Design review of the part built by this model. Coordinates are the model's own, in mm. Face numbers are marked on the shaded views. A direction names the side the tool comes from. Round coordinates to 2 decimals unless told otherwise and drop trailing zeros. Loops run counter-clockwise (first coordinate to the right, second up) from the corner with the lowest first, then second, coordinate; pieces in that order, holes last. Notation, with made-up numbers: M 22,51 L 30,51 A37 cw 30,88 Z; hole C -6.5,4.5 d4. An arc over 180 degrees is marked long. One line per item, written item: value. Start each with the question number.
Item 1: We need section B-B (x = 10.72). Write out the cut boundary in (y, z).
Item 2: Clearance check with flat-ended pins moving along their axes: pin 1 (0.8 mm diameter, centred on y = 20, z = 5, fed in from +X); pin 2 (2 mm diameter, centred on y = 20, z = 5, fed in from -X); pin 3 (6 mm diameter, centred on x = 35.5, y = 26, fed in from +Z). State where each tip first meets the part, or that it passes through.
Item 3: Mouldability with a two-part tool opening along Y and no side actions: class the marked faces 1, 2 and 3 as released by +Y, released by -Y, zero draft, split by the parting line, or undercut.
Item 4: For the marked faces 4 and 5, list the 3-axis set-ups (+Z, -Z, +X, -X, +Y, -Y) from which the entire face can be reached by the end or side of a thin tool; tool diameter is ignored.
Item 5: For line 1 along Y through (x, z) = (27.5, 6.9); line 2 along X through (y, z) = (5.5, 4.95); line 3 along Y through (x, z) = (52.5, 4.75), list the stretches that pass through material, from the lowest coordinate up.
Item 6: We need section A-A (y = 48). Write out the cut boundary in (x, z).
from build123d import *

# Parameters (mm, degrees)
SKETCH_W        = 55
SKETCH_H        = 75.8
PAD_DEPTH       = 3.6
SKETCH001_W     = 51.76
SKETCH001_H     = 74.18
PAD001_DEPTH    = 5
POCKET_DEPTH    = 7
SKETCH003_R     = 2
PAD002_DEPTH    = 7.25
SKETCH004_W     = 10
SKETCH004_H     = 2.5
POCKET001_DEPTH = 1
SKETCH005_W     = 10
SKETCH005_H     = 2.5
POCKET002_DEPTH = 1
POCKET003_DEPTH = 2.3
SKETCH007_R     = 1.6
POCKET004_DEPTH = 6.551
CHAMFER_SIZE    = 5
CHAMFER001_SIZE = 2
CHAMFER002_SIZE = 1
CHAMFER003_SIZE = 1
CHAMFER004_SIZE = 1
FILLET_R        = 3
CHAMFER005_SIZE = 0.5
CHAMFER006_SIZE = 1


with BuildPart() as part:
    # Sketch → Pad (new body)
    with BuildSketch(Plane.XY):
        with Locations((27.5, 37.9)):
            Rectangle(SKETCH_W, SKETCH_H)
    extrude(amount=PAD_DEPTH)

    # Sketch001 → Pad001 (new body)
    with BuildSketch(Plane.XY.offset(3.6)):
        with Locations((27.5, 37.09)):
            Rectangle(SKETCH001_W, SKETCH001_H)
    extrude(amount=PAD001_DEPTH)

    # Sketch002 → Pocket (cut)
    with BuildSketch(Plane.XY.offset(8.6)):
        Polygon((18.22, 1.6), (3.22, 1.6), (3.22, 72.58), (51.78, 72.58), (51.78, 1.6), (36.78, 1.6), (36.78, 14.1), (18.22, 14.1), align=None)
    extrude(amount=-POCKET_DEPTH, mode=Mode.SUBTRACT)

    # Sketch003 → Pad002 (new body)
    with BuildSketch(Plane.XY.offset(1.6)):
        with Locations((10.72, 52.58)):
            Circle(SKETCH003_R)
        with Locations((44.28, 52.58)):
            Circle(SKETCH003_R)
        with Locations((18.22, 18.6)):
            Circle(SKETCH003_R)
        with Locations((36.78, 18.6)):
            Circle(SKETCH003_R)
    extrude(amount=PAD002_DEPTH)

    # Sketch004 → Pocket001 (cut)
    with BuildSketch(Plane.YZ.offset(53.38)):
        with Locations((19, 5.35)):
            Rectangle(SKETCH004_W, SKETCH004_H)
        with Locations((57.5, 5.35)):
            Rectangle(SKETCH004_W, SKETCH004_H)
    extrude(amount=-POCKET001_DEPTH, mode=Mode.SUBTRACT)

    # Sketch005 → Pocket002 (cut)
    with BuildSketch(Plane(origin=(1.62, 0, 0), x_dir=(0, -1, 0), z_dir=(-1, 0, 0))):
        with Locations((-57.5, 5.35)):
            Rectangle(SKETCH005_W, SKETCH005_H)
        with Locations((-19, 5.35)):
            Rectangle(SKETCH005_W, SKETCH005_H)
    extrude(amount=-POCKET002_DEPTH, mode=Mode.SUBTRACT)

    # Sketch006 → Pocket003 (cut)
    with BuildSketch(Plane(origin=(0, 0, 0), x_dir=(1, 0, 0), z_dir=(0, 0, -1))):
        with BuildLine():
            Line((22, 0), (33, 0))
            Line((33, 0), (33, -5.500002))
            ThreePointArc((27.500001, -11), (31.389087, -9.389088), (33, -5.500002))
            Line((27.500001, -11), (27.499999, -11))
            ThreePointArc((22, -5.500002), (23.610913, -9.389088), (27.499999, -11))
            Line((22, -5.500002), (22, 0))
        make_face()
    extrude(amount=-POCKET003_DEPTH, mode=Mode.SUBTRACT)

    # Sketch007 → Pocket004 (cut, through all)
    with BuildSketch(Plane(origin=(0, 0, 2.3), x_dir=(1, 0, 0), z_dir=(0, 0, -1))):
        with Locations((27.5, -5.5)):
            Circle(SKETCH007_R)
    extrude(amount=-POCKET004_DEPTH, mode=Mode.SUBTRACT)

    # Chamfer
    chamfer_edges = [part.edges().sort_by_distance(p)[0] for p in [
        (18.22, 14.1, 5.1),
        (36.78, 14.1, 5.1),
    ]]
    chamfer(chamfer_edges, length=CHAMFER_SIZE)

    # Chamfer001
    chamfer001_edges = [part.edges().sort_by_distance(p)[0] for p in [
        (3.22, 72.58, 5.1),
        (51.78, 72.58, 5.1),
    ]]
    chamfer(chamfer001_edges, length=CHAMFER001_SIZE)

    # Chamfer002
    chamfer002_edges = [part.edges().sort_by_distance(p)[0] for p in [
        (3.22, 36.09, 1.6),
        (4.22, 71.58, 1.6),
        (10.72, 1.6, 1.6),
        (27.5, 72.58, 1.6),
        (18.22, 5.35, 1.6),
        (50.78, 71.58, 1.6),
        (20.72, 11.6, 1.6),
        (51.78, 36.09, 1.6),
        (27.5, 14.1, 1.6),
        (44.28, 1.6, 1.6),
        (34.28, 11.6, 1.6),
        (36.78, 5.35, 1.6),
        (8.72, 52.58, 1.6),
        (42.28, 52.58, 1.6),
        (34.78, 18.6, 1.6),
        (16.22, 18.6, 1.6),
    ]]
    chamfer(chamfer002_edges, length=CHAMFER002_SIZE)

    # Chamfer003
    chamfer003_edges = [part.edges().sort_by_distance(p)[0] for p in [
        (25.9, 5.5, 2.3),
    ]]
    chamfer(chamfer003_edges, length=CHAMFER003_SIZE)

    # Chamfer004
    chamfer004_edges = [part.edges().sort_by_distance(p)[0] for p in [
        (23.610913, 9.389088, 0),
        (31.389087, 9.389088, 0),
    ]]
    chamfer(chamfer004_edges, length=CHAMFER004_SIZE)

    # Fillet
    fillet_edges = [part.edges().sort_by_distance(p)[0] for p in [
        (1.62, 74.18, 6.1),
        (0, 75.8, 1.8),
        (0, 37.9, 0),
        (27.5, 75.8, 0),
        (53.38, 74.18, 6.1),
        (55, 37.9, 0),
        (55, 75.8, 1.8),
    ]]
    fillet(fillet_edges, radius=FILLET_R)

    # Chamfer005
    chamfer005_edges = [part.edges().sort_by_distance(p)[0] for p in [
        (1.62, 35.59, 8.6),
        (2.49868, 73.30132, 8.6),
        (27.5, 0, 8.6),
        (27.5, 74.18, 8.6),
        (53.38, 35.59, 8.6),
        (52.50132, 73.30132, 8.6),
        (51.78, 36.09, 8.6),
        (50.78, 71.58, 8.6),
        (44.28, 1.6, 8.6),
        (27.5, 72.58, 8.6),
        (36.78, 5.35, 8.6),
        (4.22, 71.58, 8.6),
        (34.28, 11.6, 8.6),
        (3.22, 36.09, 8.6),
        (27.5, 14.1, 8.6),
        (10.72, 1.6, 8.6),
        (20.72, 11.6, 8.6),
        (18.22, 5.35, 8.6),
        (25.9, 5.5, 8.6),
    ]]
    chamfer(chamfer005_edges, length=CHAMFER005_SIZE)

    # Chamfer006
    chamfer006_edges = [part.edges().sort_by_distance(p)[0] for p in [
        (43, 0, 0),
        (12, 0, 0),
    ]]
    chamfer(chamfer006_edges, length=CHAMFER006_SIZE)


solid = part.part
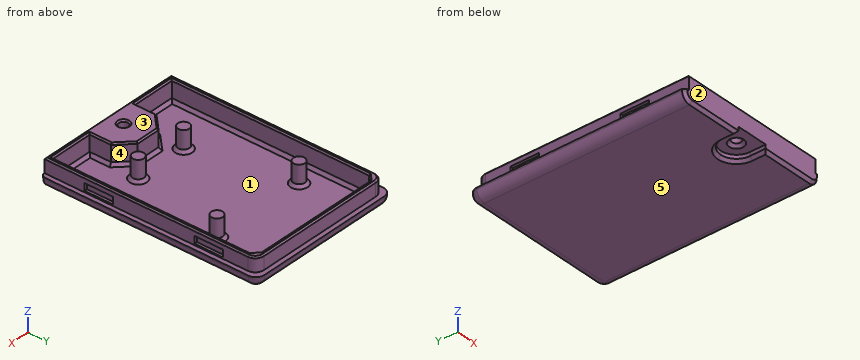
A:
1. outline: M 0,1 L 1,0 L 72.8,0 A3 ccw 75.8,3 L 75.8,3.6 L 74.18,3.6 L 74.18,8.1 L 73.68,8.6 L 73.08,8.6 L 72.58,8.1 L 72.58,2.6 L 71.58,1.6 L 55.58,1.6 L 54.58,2.6 L 54.58,8.85 L 50.58,8.85 L 50.58,2.6 L 49.58,1.6 L 2.6,1.6 L 1.6,2.6 L 1.6,8.1 L 1.1,8.6 L 0.5,8.6 L 0,8.1 Z
2. pin 1: x = 52.38
2. pin 2: x = 1.62
2. pin 3: z = 1.6
3. face 1: undercut
3. face 2: released by -Y
3. face 3: zero draft
4. face 4: +Z
4. face 5: -Z, +X, -X, +Y, -Y
5. line 1: 0 to 3.9, 7.1 to 14.1, 72.58 to 74.18
5. line 2: 1.62 to 3.22, 18.22 to 25.9, 29.1 to 36.78, 51.78 to 53.38
5. line 3: 0 to 14, 24 to 52.5, 62.5 to 73.3
6. outline: M 0,3 A3 ccw 3,0 L 52,0 A3 ccw 55,3 L 55,3.6 L 53.38,3.6 L 53.38,8.1 L 52.88,8.6 L 52.28,8.6 L 51.78,8.1 L 51.78,2.6 L 50.78,1.6 L 4.22,1.6 L 3.22,2.6 L 3.22,8.1 L 2.72,8.6 L 2.12,8.6 L 1.62,8.1 L 1.62,3.6 L 0,3.6 Z
